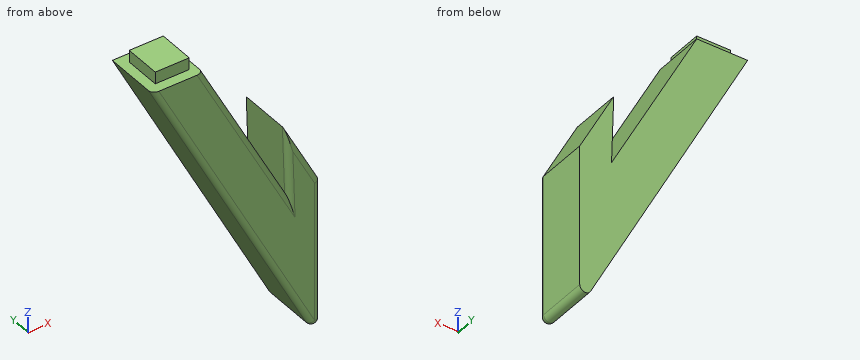
from build123d import *

# Parameters (mm, degrees)
F1_DEPTH = 10
F3_DEPTH = 2.1
F5_R     = 1


# Not quite as in the source:
# - a feature of the source that left no trace in its solid (it failed there, or was rolled back) is left out


with BuildPart() as f1:
    # F0 (on Front) → F1 (new body)
    with BuildSketch(Plane.XZ):
        Polygon((9, 0), (0, 0), (29.6767346319, -56.9180645261), (29.6767346319, -28.0180645261), (23.6665218482, -16.6037164372), (24.0578948756, -28.5973325372), align=None)
    extrude(amount=F1_DEPTH)

    # F2 (on face) → F3 (join)
    with BuildSketch(Plane.XY):
        Polygon((7.7660586685, -1.75), (1.75, -1.75), (1.75, -8.23), (7.75, -8.23), align=None)
    extrude(amount=F3_DEPTH)

    # F5
    f5_edges = [f1.edges().sort_by_distance(p)[0] for p in [
        (16.528947, -10, -14.298666),
        (23.862208, -10, -22.600524),
        (26.671628, -10, -22.31089),
        (29.676735, -10, -42.468065),
        (14.838367, -10, -28.459032),
        (29.676735, -5, -56.918065),
    ]]
    fillet(f5_edges, radius=F5_R)


solid = f1.part
The model under review builds one solid part; all positions refer to its coordinate system, in mm. Give positions to 0.01 mm unless a question says otherwise; leave off trailing zeros. Order: outer loops, then holes, each group sorted by start corner. A loop starts at its lowest first (then second) coordinate and runs counter-clockwise, first axis right, second up. Notation, with made-up numbers: (80, 29) -> (90, 29) arc R10 ccw to (90, 34) -> close; hole circle Ø8 at (-15, 84). An arc over 180 degrees is marked (long way). Write item = value, one per line. Start each with the question number.
(1) For pin 1 Ø2 at (y, z) = (-7, -18) entering from +X; pin 2 Ø5 at (y, z) = (-6, -43) entering from -X; pin 3 Ø1 at (y, z) = (-5.5, -20.5) entering from +X, all flat-tipped, find the tip position at first contact; note any pin that passes through.
(2) Take a section at A-A (y = -4). Write out the cut boundary in (x, z), plus the area to 3 significant figures.
(3) For L1, parallel to X at y = -5.75, z = -18.5 (3 decimals); L2, parallel to X at y = -1, z = -20; L3, parallel to X at y = -5.5, z = -45.5, list the stretches that pass through material, from the lowest coordinate up. Write a range as from..to.
(4) Take a section at B-B (y = -6.25). Write out the cut boundary in (x, z).
Returned:
q1.pin_1 = 24.93
q1.pin_2 = 21.12
q1.pin_3 = 25.98
q2.outline = (0, 0) -> (27.79, -53.3) arc R1 ccw to (29.68, -52.84) -> (29.68, -28.02) -> (23.67, -16.6) -> (24.06, -28.6) -> (9, 0) -> (7.76, 0) -> (7.76, 2.1) -> (1.75, 2.1) -> (1.75, 0) -> close
q2.area = 514 mm²
q3.L1 = 9.646..18.741, 23.728..24.665
q3.L2 = 10.43..19.53, 23.78..25.45
q3.L3 = 23.72..29.68
q4.outline = (0, 0) -> (27.79, -53.3) arc R1 ccw to (29.68, -52.84) -> (29.68, -28.02) -> (23.67, -16.6) -> (24.06, -28.6) -> (9, 0) -> (7.75, 0) -> (7.75, 2.1) -> (1.75, 2.1) -> (1.75, 0) -> close
